Part model, mm, in its own coordinate system. Round coordinates to 2 decimals unless told otherwise and drop trailing zeros. Loops run counter-clockwise (first coordinate to the right, second up) from the corner with the lowest first, then second, coordinate; pieces in that order, holes last. Notation, with made-up numbers: (43.25, -37.5) - (62.25, -37.5) arc R20 cw to (62.25, -7.5) - close; hole circle Ø9 at (42.25, 63). An arc over 180 degrees is marked (long way). Write each question's results on one line, items separated by ' | '. Start each with the question number.
(1) Drill centre lines: L1, parallel to X at y = 4.8, z = -37.5; L2, parallel to X at y = 4.4, z = -16; L3, parallel to Z at x = -31.5, y = 1.9. Where is each one in solid material? Low to high.
(2) Cut at A-A, the plane z = 0. List the corners of the cut face in (x, y).
(3) Cut at B-B, the plane z = -25. List the corners of the cut face in (x, y), then the cut area to 4 significant figures.
(4) Flat gauge pins, fed straight in: P1, Ø4, axis at x = -37.28, z = -37.37, coming from the +Y side; P2, Ø3, axis at x = -59, y = 2.5, coming from the -Z side; P3, Ø1, axis at y = 1.5, z = -57, coming from the +X side; P4, Ø1.5, axis at y = 1, z = -36, coming from the -X side. Where does each tip first touch, or does it go through?
(5) Cut at D-D, the plane x = -90. List the corners of the cut face in (y, z), then the cut area to 3 significant figures.
(6) Cut at C-C, the plane y = 2.85. List the corners of the cut face in (x, z), then the cut area to 3 significant figures.
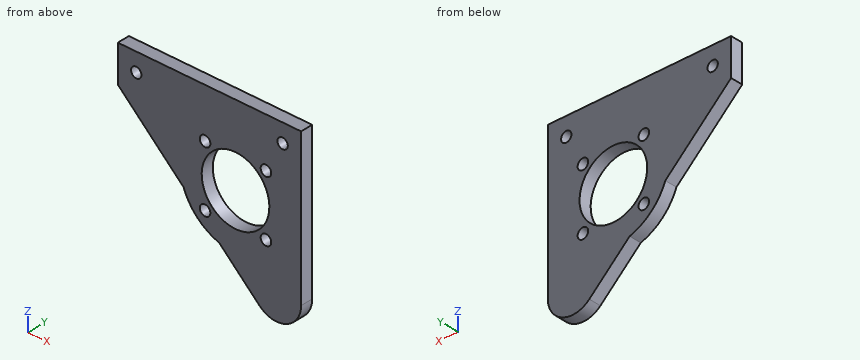
from build123d import *

# Parameters (mm, degrees)
SKETCH_1_R          = 2.1
SKETCH_1_R_2        = 2.15
SKETCH_1_R_3        = 13.75
EXTRUDE_1_DEPTH     = 5
CUT_EXTRUDE_1_DEPTH = 5
FILLET_1_R          = 10


with BuildPart() as part:
    # ｽｹｯﾁ1 → ﾎﾞｽ - 押し出し1 (new body)
    with BuildSketch(Plane(origin=(0, 0, 0), x_dir=(1, 0, 0), z_dir=(0, 1, 0))):
        with BuildLine():
            Line((5, -7.5), (5, 0))
            Line((5, 0), (5, 90))
            Line((5, 90), (5, 95))
            Line((5, 95), (-5, 95))
            Line((-5, 95), (-56.263686619, 46.507323468))
            ThreePointArc((-56.263686619, 46.507323468), (-65.116217602, 41.345539381), (-70.761470202, 32.793203863))
            Line((-70.761470202, 32.793203863), (-97.5, 7.5))
            Line((-97.5, 7.5), (-97.5, -7.5))
            Line((-97.5, -7.5), (0, -7.5))
            Line((0, -7.5), (5, -7.5))
        make_face()
        with Locations(Location((-90, 0, 0), (0, 0, 270))):
            Circle(SKETCH_1_R, mode=Mode.SUBTRACT)
        with Locations(Location((-62.02858956, 12.625631329, 0), (0, 0, 270))):
            Circle(SKETCH_1_R_2, mode=Mode.SUBTRACT)
        with Locations(Location((-49.654220889, 25, 0), (0, 0, 270))):
            Circle(SKETCH_1_R_3, mode=Mode.SUBTRACT)
        with Locations(Location((-62.02858956, 37.374368671, 0), (0, 0, 270))):
            Circle(SKETCH_1_R_2, mode=Mode.SUBTRACT)
        with Locations(Location((-30.5, 0, 0), (0, 0, 270))):
            Circle(SKETCH_1_R, mode=Mode.SUBTRACT)
        with Locations(Location((-37.279852219, 12.625631329, 0), (0, 0, 270))):
            Circle(SKETCH_1_R_2, mode=Mode.SUBTRACT)
        with Locations(Location((0, 0, 0), (0, 0, 270))):
            Circle(SKETCH_1_R, mode=Mode.SUBTRACT)
        with Locations(Location((-37.279852219, 37.374368671, 0), (0, 0, 270))):
            Circle(SKETCH_1_R_2, mode=Mode.SUBTRACT)
        with Locations(Location((0, 90, 0), (0, 0, 270))):
            Circle(SKETCH_1_R_2, mode=Mode.SUBTRACT)
    extrude(amount=EXTRUDE_1_DEPTH)

    # ｽｹｯﾁ2 → ｶｯﾄ - 押し出し1 (cut)
    with BuildSketch(Plane(origin=(0, 5, 0), x_dir=(1, 0, 0), z_dir=(0, 1, 0))):
        Polygon((-23, -7.5), (-23, 77.972972973), (-5, 95), (5, 95), (5, -7.5), align=None)
    extrude(amount=-CUT_EXTRUDE_1_DEPTH, mode=Mode.SUBTRACT)

    # ﾌｨﾚｯﾄ1
    fillet_1_edges = [part.edges().sort_by_distance(p)[0] for p in [
        (-23, 2.5, -77.972972973),
    ]]
    fillet(fillet_1_edges, radius=FILLET_1_R)


solid = part.part
A:
1) L1: -68.36 to -64.17, -59.88 to -55.38, -43.93 to -39.43, -35.13 to -23 | L2: -88.51 to -60.05, -39.26 to -23 | L3: -64.64 to -1.85, 1.85 to 7.5
2) outline: (-97.5, 0) - (-92.1, 0) - (-92.1, 5) - (-97.5, 5) - close; (-87.9, 0) - (-32.6, 0) - (-32.6, 5) - (-87.9, 5) - close; (-28.4, 0) - (-23, 0) - (-23, 5) - (-28.4, 5) - close
3) outline: (-79, 0) - (-63.4, 0) - (-63.4, 5) - (-79, 5) - close; (-35.9, 0) - (-23, 0) - (-23, 5) - (-35.9, 5) - close | area: 142.5 mm2
4) P1: through | P2: z = -46.09 | P3: x = -23.15 | P4: x = -69.68
5) outline: (0, -14.59) - (5, -14.59) - (5, -2.1) - (0, -2.1) - close; (0, 2.1) - (5, 2.1) - (5, 7.5) - (0, 7.5) - close | area: 89.5 mm2
6) outline: (-97.5, -7.5) - (-70.76, -32.79) arc R22.5 ccw to (-56.26, -46.51) - (-39.87, -62.01) arc R10 ccw to (-23, -54.75) - (-23, 7.5) - (-97.5, 7.5) - close; hole circle Ø4.2 at (-90, 0); hole circle Ø4.3 at (-62.03, -37.37); hole circle Ø4.3 at (-62.03, -12.63); hole circle Ø27.5 at (-49.65, -25); hole circle Ø4.3 at (-37.28, -37.37); hole circle Ø4.3 at (-37.28, -12.63); hole circle Ø4.2 at (-30.5, 0) | area: 2,980 mm2
